Verification items for the finished model (mm, model axes). Give positions to 0.01 mm unless a question says otherwise; leave off trailing zeros. Write each loop counter-clockwise with the first axis right and the second up, starting at its lowest first coordinate (ties: lowest second). Pieces come first, ordered by that corner, then holes. Notation, with made-up numbers: (51, 88.5) - (94, 88.5) arc R12 cw to (94, 110.5) - close; hole circle Ø5 at (1, 14). An arc over 180 degrees is marked (long way). Answer as a JSON object with one key per item and string values. Group by question number.
Item 1: Go/stop test with flat-tipped pins: pin 1 (1 mm diameter, centred on x = -2, y = 27, fed in from -Z); pin 2 (1 mm diameter, centred on y = 34, z = 2.5, fed in from +X); pin 3 (2 mm diameter, centred on x = 1.5, y = 9.5, fed in from -Z). Record where each tip stops, or that it passes through.
Item 2: Sectioned sample at B-B, the plane z = 0. Record the boundary of the cut face in (x, y), and give its area (3 significant figures).
Item 3: Scan lines: line 1 along X through (y, z) = (30, 0); line 2 along Z through (x, y) = (0, 20.5); line 3 along X through (y, z) = (13, 0.75). Record each from-to range of solid material in increasing order. Write a range as [from, to].
Item 4: Sectioned sample at A-A, the plane y = 21. Record the boundary of the cut face in (x, z), and give its area (3 significant figures).
```python
from build123d import *

# Parameters (mm, degrees)
SKETCH_1_R      = 1.5
EXTRUDE_1_DEPTH = 60


with BuildPart() as part:
    # Эскиз1 → Бобышка-Вытянуть1 (new body)
    with BuildSketch(Plane(origin=(0, 0, 0), x_dir=(1, 0, 0), z_dir=(0, 1, 0))):
        Polygon((0, 3.175426481), (-2.75, 1.58771324), (-2.75, -1.58771324), (0, -3.175426481), (2.75, -1.58771324), (2.75, 1.58771324), align=None)
        Circle(SKETCH_1_R, mode=Mode.SUBTRACT)
    extrude(amount=EXTRUDE_1_DEPTH)

    # Эскиз3 → Вырез-Повернуть1 (revolve, cut)
    with BuildSketch(Plane(origin=(0, 0, 0), x_dir=(0, 0, -1), z_dir=(1, 0, 0))):
        Polygon((-8.378043736, 3.328738228), (-8.378043736, 0), (-2.6125, 0), align=None)
        Polygon((-11.931875613, 60), (-2.6125, 60), (-11.931875613, 54.619455981), align=None)
    revolve(axis=Axis((0, 60, 0), (0, -1, 0)), mode=Mode.SUBTRACT)


solid = part.part
```
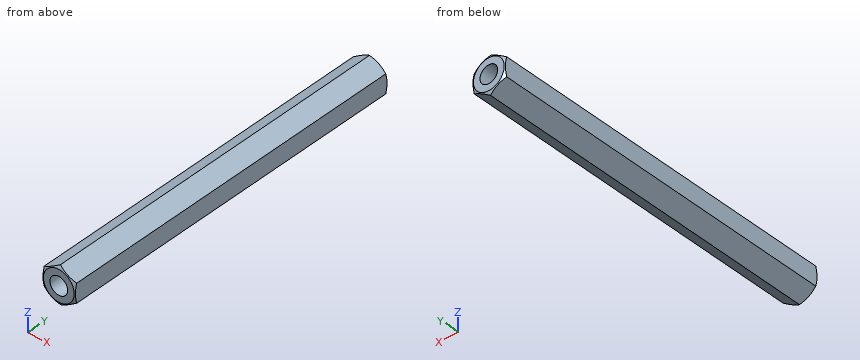
Geometry check:
{
 "1": {"pin 1": "z = -2.31", "pin 2": "x = 2.04", "pin 3": "z = -2.89"},
 "2": {"outline": "(-2.75, 0.08) - (-2.61, 0) - (-1.5, 0) - (-1.5, 60) - (-2.61, 60) - (-2.75, 59.92) - close; (1.5, 0) - (2.61, 0) - (2.75, 0.08) - (2.75, 59.92) - (2.61, 60) - (1.5, 60) - close", "area": "150 mm^2"},
 "3": {"line 1": "[-2.75, -1.5], [1.5, 2.75]", "line 2": "[-3.18, -1.5], [1.5, 3.18]", "line 3": "[-2.75, -1.3], [1.3, 2.75]"},
 "4": {"outline": "(-2.75, -1.59) - (0, -3.18) - (2.75, -1.59) - (2.75, 1.59) - (0, 3.18) - (-2.75, 1.59) - close; hole circle Ø3 at (0, 0)", "area": "19.1 mm^2"}
}
